Source: CAD feature listing. Evaluate the final solid. Frame: model axes, mm. Round coordinates to 2 decimals unless told otherwise and drop trailing zeros. Order: outer loops, then holes, each group sorted by start corner. A loop starts at its lowest first (then second) coordinate and runs counter-clockwise, first axis right, second up. Notation, with made-up numbers: (-14.75, 63.25) - (39.25, 63.25) arc R30 ccw to (39.25, 93.25) - close; hole circle Ø1 at (3.25, 50). An arc over 180 degrees is marked (long way). Use one line per item in the form item = value. Start each with the question number.
Q1. Pin query (flat end, axial travel): pin 1 Ø10 at (y, z) = (-64, 29.5) entering from +X; pin 2 Ø1.5 at (y, z) = (-91.5, 27.5) entering from +X; pin 3 Ø2 at (y, z) = (-196, 33) entering from -X. Return the tip coordinate at first contact, or that it passes through.
Q2. Cut plane D-D, the plane x = 15. Return the cut outline in (y, z).
Q3. Cut plane C-C, the plane z = 15. Return the cut outline in (x, y).
Q4. Draft query along X for faces 1 (the cylindrical face through (-5.07, -125.22, 14.6)), 2 (the flat face through (-8.909, -125.222, 40.846)), 3 (the flat face through (26.446, -125, -5)). Return one class per face: released by +X, released by -X, zero draft, split by the parting line, or undercut.
Q5. Ray query, line 1 (X direction, y = -83, z = 36.5); line 2 (Z direction, x = 15.5, y = -157.5); line 3 (Z direction, x = -11.5, y = -119). Return the intervals inside material, ascending. Write a range as [from, to].
Q6. Cut plane B-B, the plane y = -33. Return the cut outline in (x, z), and give its area (3 significant figures).
Q7. Cut plane A-A, the plane x = -14. Return the cut outline in (y, z), and give its area (3 significant figures).
from build123d import *

# Parameters (mm, degrees)
F1_DEPTH = 254
F3_D     = 25.4


with BuildPart() as f1:
    # F0 (on Front) → F1 (new body)
    with BuildSketch(Plane.XZ):
        Polygon((0, 49.849775), (-26.433898, 23.133671), (-26.433898, -31.603329), (26.446328, -31.603329), (26.446328, 23.133671), align=None)
    extrude(amount=F1_DEPTH)

    # F3 (through all)
    with Locations(Plane.XZ.offset(254)):
        with Locations((-17.007671, 18.930277)):
            Hole(F3_D / 2)


solid = f1.part
Completed:
q1.pin_1 = 25.09
q1.pin_2 = 22.87
q1.pin_3 = -17.66
q2.outline = (-254, -31.6) - (0, -31.6) - (0, 34.7) - (-254, 34.7) - close
q3.outline = (-4.93, -254) - (26.45, -254) - (26.45, 0) - (-4.93, 0) - close
q4.face_1 = undercut
q4.face_2 = released by -X
q4.face_3 = released by +X
q5.line_1 = [-13.21, 13.21]
q5.line_2 = [-31.6, 34.19]
q5.line_3 = [-31.6, 7.49], [30.37, 38.23]
q6.outline = (-26.43, -31.6) - (26.45, -31.6) - (26.45, 23.13) - (0, 49.85) - (-18.07, 31.59) arc R12.7 cw (long way) to (-26.43, 10.42) - close
q6.area = 3,160 mm2
q7.outline = (-254, -31.6) - (0, -31.6) - (0, 6.59) - (-254, 6.59) - close; (-254, 31.27) - (0, 31.27) - (0, 35.7) - (-254, 35.7) - close
q7.area = 10,800 mm2
